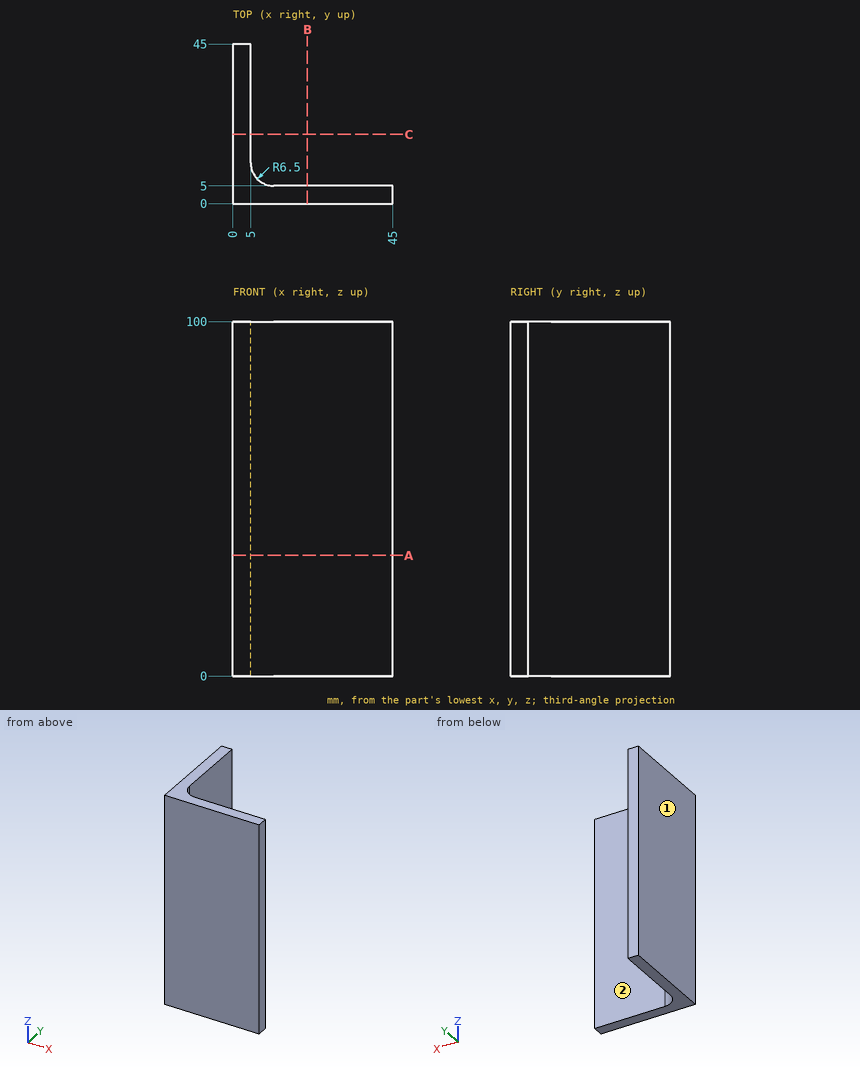
Can you work these out from the drawing? Everything is in mm from the part's minimum corner. A direction names the side the tool comes from. Round coordinates to 2 decimals unless told otherwise and drop trailing zeros. Write each loop counter-clockwise with the first axis right and the second up, starting at its lowest first coordinate (ties: lowest second). Pieces come first, ordered by that corner, then holes. Notation, with made-up numbers: (-13.75, 49.25) - (33.25, 49.25) arc R15 cw to (33.25, 75.25) - close; hole circle Ø7 at (62, 2). An arc over 180 degrees is marked (long way). Write each question's results on one line, items separated by ' | '. Start each with the question number.
1) Which directions (+Z, -Z, +X, -X, +Y, -Y) give clear straight access to the entire face, cutting with the end or side of a thin tool? Please do the marked faces 1 and 2.
2) For pin 1 Ø4 at (x, z) = (39, 79.5) entering from +Y; pin 2 Ø1 at (y, z) = (17, 28) entering from +X, each with a flat end and sliding along its axis, tell me the tip position at first contact or that it passes through.
3) Suppose I cut it at A-A (z = 34). List the corners of the cut face in (x, y) for me.
4) Please list where these lines run through material, in increasing order: line 1 (Y direction, x = 15, z = 58); line 2 (Y direction, x = 10.5, z = 55).
5) Suppose I cut it at B-B (x = 21). List the corners of the cut face in (y, z) for me.
Here are the results:
1) face 1: +Z, -Z, -X, +Y, -Y | face 2: +Z, -Z, +X, +Y
2) pin 1: stops at y = 5 | pin 2: stops at x = 5
3) outline: (0, 0) - (45, 0) - (45, 5) - (11.5, 5) arc R6.5 cw to (5, 11.5) - (5, 45) - (0, 45) - close
4) line 1: y = 0 to 5 | line 2: y = 0 to 5.08
5) outline: (0, 0) - (5, 0) - (5, 100) - (0, 100) - close
